Could you check a few things on this model? Use its own coordinates, in mm. Face numbers are marked on the shaded views. Coordinates: 2 decimals unless noted, no trailing zeros. Order: outer loops, then holes, each group sorted by start corner. A loop starts at its lowest first (then second) coordinate and runs counter-clockwise, first axis right, second up. Notation, with made-up numbers: (43, -10) -> (59, -10) arc R23 cw to (59, 27) -> close; hole circle Ø3 at (33, -10). An arc over 180 degrees is marked (long way). Use a Markdown table: item, result. Add a question column.
1) If we section it at C-C (y = -7.5): Write out the boundary of the cut face in (x, z).
2) If I drill on L1, parallel to Z at x = -3.4, y = -17; L2, parallel to Z at x = -3.8, y = -10.25; L3, parallel to X at y = 2, z = -15.5, over which ranges is the centre line in solid material (lowest first)? Write a range as [from, to].
3) If we section it at A-A (y = 0): Write out the boundary of the cut face in (x, z).
4) If we section it at D-D (x = -4.9): Give the number of separate pieces and of enclosed holes in the cut face, plus the area to 3 significant figures.
5) Thinking about a two-plate mould opening in Y: for the marked faces 1, 2 and 3, which applies, +Y half, -Y half, draft (parallel to the pull), parting line (faces both ways), or undercut?
6) Will these pins go through, and if not, where does the flat tip stop? pin 1 Ø1 at (x, z) = (-4.5, 11.5) entering from -Y; pin 2 Ø1.6 at (y, z) = (10.25, -17.75) entering from -X; pin 3 Ø2 at (x, y) = (-2, 1) entering from +Z; pin 4 Ø1 at (x, z) = (-2.5, -19) entering from +Y.
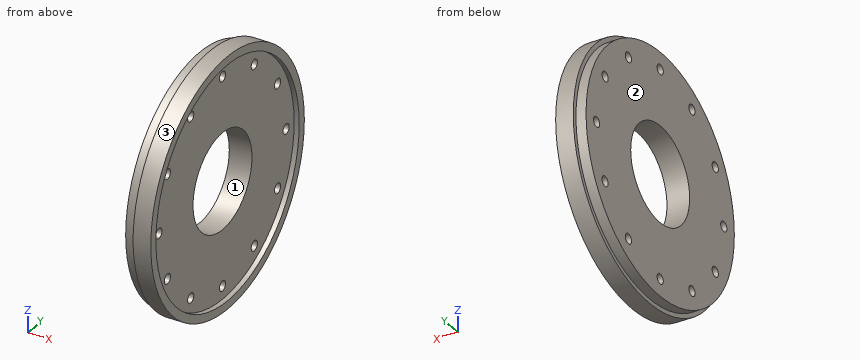
Autodesk Inventor part; units mm, degrees
ref_plane "YZ Plane" through (0, 0, 0) normal (1, 0, 0) x (0, 1, 0)
ref_plane "XZ Plane" through (0, 0, 0) normal (0, 1, 0) x (-1, 0, 0)
ref_plane "XY Plane" through (0, 0, 0) normal (0, 0, 1) x (1, 0, 0)
sketch "Sketch1" plane through (0, 0, 0) normal (0, 0, 1) x (1, 0, 0)
  line L0 (-6.6, 0) -> (1.1, 0) construction
  line L1 (0, -4.95) -> (0, 29.7) construction
  line L2 (-1, 9.5) -> (-1, 23.1)
  line L3 (-1, 23.1) -> (0, 23.1)
  line L4 (0, 23.1) -> (0, 24.75)
  line L5 (0, 24.75) -> (-3.5, 24.75)
  line L6 (-3.5, 24.75) -> (-3.5, 23.9)
  line L7 (-3.5, 23.9) -> (-5.5, 23.9)
  line L8 (-5.5, 23.9) -> (-5.5, 9.5)
  line L9 (-5.5, 9.5) -> (-1, 9.5)
  point P0 (0, 0)
  dimension "d0" = 49.5
  dimension "d1" = 47.8
  dimension "d2" = 19
  dimension "d3" = 2
  dimension "d4" = 1
  dimension "d5" = 5.5
  dimension "d6" = 46.2
revolve "Revolution1" add sketch "Sketch1" angle 360 about axis through (-10, 0, 0) along (1, 0, 0)
sketch "Sketch2" plane through (-1, 0, 0) normal (1, 0, 0) x (0, 0, -1)
  line L0 (0, -34.65) -> (0, 34.65)
  line L1 (34.65, 0) -> (-34.65, 0)
  point P0 (0, 0)
  point P1 (-20.5, 0)
  dimension "d8" = 20.5
hole "Hole1" at (-1, 0, 20.5) direction (-1, 0, 0) diameter 2 end through all
pattern_circular "Circular Pattern1" count 12 over 360 about axis through (-10, 0, 0) along (1, 0, 0) of "Hole1"
thread "Thread1"
properties part number "P302Base" material "ABS Plastic"
Answer sheet:
| question | item | result |
|---|---|---|
| 1 | outline | (-5.5, -22.69) -> (-3.5, -22.69) -> (-3.5, -23.59) -> (0, -23.59) -> (0, -21.85) -> (-1, -21.85) -> (-1, -5.83) -> (-5.5, -5.83) -> close; (-5.5, 5.83) -> (-1, 5.83) -> (-1, 21.85) -> (0, 21.85) -> (0, 23.59) -> (-3.5, 23.59) -> (-3.5, 22.69) -> (-5.5, 22.69) -> close |
| 2 | L1 | [-17.99, -10.91], [-9.59, 9.59], [10.91, 17.99] |
| 2 | L2 | [-21.59, -18.75], [-16.75, 16.75], [18.75, 21.59] |
| 2 | L3 | [-5.5, -1] |
| 3 | outline | (-5.5, -23.9) -> (-3.5, -23.9) -> (-3.5, -24.75) -> (0, -24.75) -> (0, -23.1) -> (-1, -23.1) -> (-1, -21.5) -> (-5.5, -21.5) -> close; (-5.5, -19.5) -> (-1, -19.5) -> (-1, -9.5) -> (-5.5, -9.5) -> close; (-5.5, 9.5) -> (-1, 9.5) -> (-1, 19.5) -> (-5.5, 19.5) -> close; (-5.5, 21.5) -> (-1, 21.5) -> (-1, 23.1) -> (0, 23.1) -> (0, 24.75) -> (-3.5, 24.75) -> (-3.5, 23.9) -> (-5.5, 23.9) -> close |
| 4 | separate pieces | 1 |
| 4 | enclosed holes | 13 |
| 4 | area | 1,470 mm2 |
| 5 | face 1 | undercut |
| 5 | face 2 | draft |
| 5 | face 3 | parting line |
| 6 | pin 1 | y = -21.22 |
| 6 | pin 2 | through |
| 6 | pin 3 | z = 24.75 |
| 6 | pin 4 | y = 16.44 |
